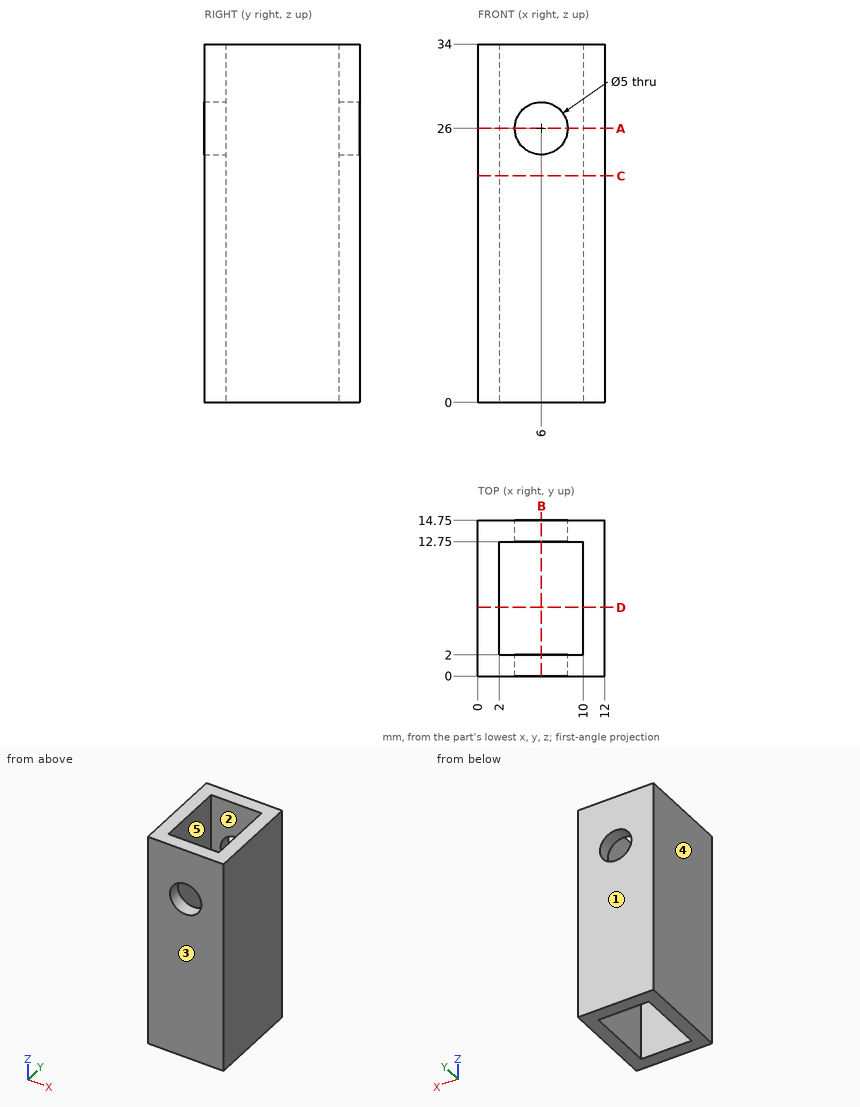
Answer from the drawing. Dimensions are ordinates in mm from the lowest x, y and z of the part. A direction names the side the tool comes from. Give positions to 0.01 mm unless a question says otherwise; leave off trailing zeros. Order: outer loops, then holes, each group sorted by start corner. A loop starts at its lowest first (then second) coordinate and runs counter-clockwise, first axis right, second up. Notation, with made-up numbers: (78.5, 35) - (135.5, 35) arc R26 cw to (135.5, 52) - close; hole circle Ø2 at (-12, 16). An arc over 180 degrees is marked (long way). One line per item, written item: value. Start each with the question number.
1. For a pull along Y with two mould halves and no side action, classify the marked faces 3, 4 and 5 as released by +Y, released by -Y, zero draft, split by the parting line, or undercut.
2. Section D-D, the plane y = 6.5 is taken. Write down the section's boundary in (x, z).
3. This flat-tipped pin is pushed along its axis until it touches: pin 1 Ø2 at (x, z) = (6.5, 26) entering from -Y. Where does it stop, or does it pass through?
4. Section A-A, the plane z = 26 is taken. Write down the section's boundary in (x, y), then the cut area to 3 significant figures.
5. Consider line 1 (X direction, y = 2.5, z = 25); line 2 (Y direction, x = 2.75, z = 6); line 3 (Z direction, x = 6, y = 0.9). Determine where each line is inside the solid, lowest interval first.
6. Which of the six approach directions +Z, -Z, +X, -X, +Y, -Y give full straight-line access (tool end or side, diameter ignored) to the marked faces 1 and 2?
7. Section B-B, the plane x = 6 is taken. Write down the section's boundary in (y, z).
8. Section C-C, the plane z = 21.5 is taken. Write down the section's boundary in (x, y).
Filled sheet:
1. face 3: released by -Y
1. face 4: zero draft
1. face 5: undercut
2. outline: (0, 0) - (2, 0) - (2, 34) - (0, 34) - close; (10, 0) - (12, 0) - (12, 34) - (10, 34) - close
3. pin 1: through
4. outline: (0, 0) - (3.5, 0) - (3.5, 2) - (2, 2) - (2, 12.75) - (3.5, 12.75) - (3.5, 14.75) - (0, 14.75) - close; (8.5, 0) - (12, 0) - (12, 14.75) - (8.5, 14.75) - (8.5, 12.75) - (10, 12.75) - (10, 2) - (8.5, 2) - close
4. area: 71.0 mm²
5. line 1: 0 to 2, 10 to 12
5. line 2: 0 to 2, 12.75 to 14.75
5. line 3: 0 to 23.5, 28.5 to 34
6. face 1: +Z, -Z, +X, -X, +Y
6. face 2: +Z, -Z
7. outline: (0, 0) - (2, 0) - (2, 23.5) - (0, 23.5) - close; (0, 28.5) - (2, 28.5) - (2, 34) - (0, 34) - close; (12.75, 0) - (14.75, 0) - (14.75, 23.5) - (12.75, 23.5) - close; (12.75, 28.5) - (14.75, 28.5) - (14.75, 34) - (12.75, 34) - close
8. outline: (0, 0) - (12, 0) - (12, 14.75) - (0, 14.75) - close; hole (2, 2) - (10, 2) - (10, 12.75) - (2, 12.75) - close
